```python
from build123d import *

# Parameters (mm, degrees)
SKETCH1_R           = 23.5
SKETCH1_R_2         = 15
BOSS_EXTRUDE1_DEPTH = 8
CUT_EXTRUDE1_START  = -8.633931
SKETCH3_R           = 2
CUT_EXTRUDE1_DEPTH  = 8.633931
CIRPATTERN1_COUNT   = 2
CIRPATTERN1_ANGLE   = 90


with BuildPart() as part:
    # Sketch1 → Boss-Extrude1 (new body)
    with BuildSketch(Plane.XY):
        Circle(SKETCH1_R)
        Circle(SKETCH1_R_2, mode=Mode.SUBTRACT)
    extrude(amount=BOSS_EXTRUDE1_DEPTH)

    # Sketch3 → Cut-Extrude1 (cut)
    with BuildSketch(Plane(origin=(0, 23.5, 8), x_dir=(1, 0, 0), z_dir=(0, 1, 0)).offset(CUT_EXTRUDE1_START)):
        with Locations((0, 4)):
            Circle(SKETCH3_R)
    cut_extrude1 = extrude(amount=CUT_EXTRUDE1_DEPTH, mode=Mode.SUBTRACT)

    # CirPattern1: Cut-Extrude1 ×2 about axis
    cirpattern1_axis = Axis((0, 0, 8), (0, 0, 1))
    for i in range(1, CIRPATTERN1_COUNT):
        add(cut_extrude1.rotate(cirpattern1_axis, i * CIRPATTERN1_ANGLE / (CIRPATTERN1_COUNT - 1)), mode=Mode.SUBTRACT)


solid = part.part
```
For this review, take the finished solid that the model builds, in its own axes (mm). A direction names the side the tool comes from. Coordinates: 2 decimals unless noted, no trailing zeros. Loops run counter-clockwise (first coordinate to the right, second up) from the corner with the lowest first, then second, coordinate; pieces in that order, holes last. Notation, with made-up numbers: (63, 29.5) - (112, 29.5) arc R8 cw to (112, 42.5) - close; hole circle Ø9 at (56, 75). An arc over 180 degrees is marked (long way). Use one line per item in the form item = value. Start each with the question number.
1) Take a section at C-C (x = 5). State the section outline as (y, z) points, plus the area to 3 significant figures.
2) Take a section at B-B (y = 0). State the section outline as (x, z) points, plus the area to 3 significant figures.
3) For pin 1 (1 mm diameter, centred on y = 2.5, z = 7, fed in from +X); pin 2 (1 mm diameter, centred on x = -18.5, z = 3, fed in from -Y); pin 3 (1.5 mm diameter, centred on x = -1, z = 6, fed in from -Y); pin 4 (24 mm diameter, centred on x = 0, y = 0, fed in from -Z), all flat-tipped, find the tip position at first contact; note any pin that passes through.
4) Draft analysis for pull direction Z (two halves, no side actions). For faces 1 (the face through (-0.3, -15.3, 0)), 2 (the face through (-19.123, 0.923, 5.774)), 3 (the face through (-0.3, -15.3, 8)), state which applies: released by +Z, released by -Z, zero draft, split by the parting line, or undercut.
5) Take a section at D-D (z = 3.25). State the section outline as (x, y) points, plus the area to 3 significant figures.
6) To check wall thickness, follow probe 1 along Z at (x, y) = (0, 17); probe 2 along X at (y, z) = (10.5, 7); probe 3 along Y at (x, z) = (3.5, 5.25). State the ranges of each line that lie inside material, in increasing order. Write a range as from..to.
7) For faces 4 (the face through (0, 19, 6)), 5 (the face through (21.71, -9, 3.94)), list the 3-axis set-ups (+Z, -Z, +X, -X, +Y, -Y) from which the entire face can be reached by the end or side of a thin tool; tool diameter is ignored.
8) Take a section at A-A (x = 0). State the section outline as (y, z) points.
From the geometry:
q1.outline = (-22.96, 0) - (-14.14, 0) - (-14.14, 8) - (-22.96, 8) - close; (14.14, 0) - (22.96, 0) - (22.96, 8) - (14.14, 8) - close
q1.area = 141 mm2
q2.outline = (-23.5, 0) - (-15, 0) - (-15, 2) - (-23.5, 2) - close; (-23.5, 6) - (-15, 6) - (-15, 8) - (-23.5, 8) - close; (15, 0) - (23.5, 0) - (23.5, 8) - (15, 8) - close
q2.area = 102 mm2
q3.pin_1 = 23.41
q3.pin_2 = -15.11
q3.pin_3 = -23.5
q3.pin_4 = through
q4.face_1 = released by -Z
q4.face_2 = undercut
q4.face_3 = released by +Z
q5.outline = (-23.43, -1.85) arc R23.5 ccw (long way) to (1.85, 23.43) - (1.85, 14.88) arc R15 cw (long way) to (-14.88, -1.85) - close; (-23.43, 1.85) - (-14.88, 1.85) arc R15 cw to (-1.85, 14.88) - (-1.85, 23.43) arc R23.5 ccw to start
q5.area = 965 mm2
q6.probe_1 = 0..2, 6..8
q6.probe_2 = -21.02..-10.71, 10.71..21.02
q6.probe_3 = -23.24..-14.59, 14.59..23.24
q7.face_4 = +Y
q7.face_5 = +Z, -Z
q8.outline = (-23.5, 0) - (-15, 0) - (-15, 8) - (-23.5, 8) - close; (15, 0) - (23.5, 0) - (23.5, 2) - (15, 2) - close; (15, 6) - (23.5, 6) - (23.5, 8) - (15, 8) - close
